CAD build for the part. Positions are in the model's coordinates, mm. A direction names the side the tool comes from. Round coordinates to 2 decimals unless told otherwise and drop trailing zeros.
from build123d import *

# Parameters (mm, degrees)
F0_R            = 19.05
F1_DEPTH        = 3.175
F3_DEPTH        = 6.35
F3_COPIES_COUNT = 16
F4_R            = 0.508
F5_R            = 6.35
F6_DEPTH        = 6.35


# Not quite as in the source:
# - a pattern or mirror of a feature is missing from the dataset's text; its kind, count and spacing are read off the source's solid


with BuildPart() as f1:
    # F0 (on Right) → F1 (new body, symmetric)
    with BuildSketch(Plane.YZ):
        Circle(F0_R)
    extrude(amount=F1_DEPTH, both=True)

    # F2 (on face) → F3 (cut, through all)
    with BuildSketch(Plane.YZ.offset(3.175)):
        with BuildLine():
            ThreePointArc((7.5322043505, 17.4976683482), (5.7520331342, 19.7340330411), (3.0490465261, 18.8044094638))
            Line((3.0490465261, 18.8044094638), (3.4766055202, 15.489636505))
            ThreePointArc((3.4766055202, 15.489636505), (4.4423475568, 15.2407733788), (5.3905576771, 14.931761883))
            Line((5.3905576771, 14.931761883), (7.5322043505, 17.4976683482))
        make_face()
    f3 = extrude(amount=-F3_DEPTH, mode=Mode.SUBTRACT)

    # F3_copies: F3 ×16 about axis
    f3_copies_axis = Axis((0, 0, 0), (1, 0, 0))
    for i in range(1, F3_COPIES_COUNT):
        add(f3.rotate(f3_copies_axis, i * 360 / F3_COPIES_COUNT), mode=Mode.SUBTRACT)

    # F4
    f4_edges = [f1.edges().sort_by_distance(p)[0] for p in [
        (0, 3.476606, 15.489637),
        (0, 5.390558, 14.931762),
        (0, 3.049047, 18.804409),
        (0, 7.532204, 17.497668),
        (0, 10.013088, 16.206189),
        (0, 9.139592, 12.980119),
        (0, 10.694364, 11.732272),
        (0, 13.654917, 13.283288),
        (0, 15.452727, 11.140724),
        (0, 13.411158, 8.494496),
        (0, 14.37005, 6.74665),
        (0, 17.698793, 7.046647),
        (0, 18.539829, 4.379184),
        (0, 15.640997, 2.715663),
        (0, 15.858026, 0.733912),
        (0, 19.048187, -0.262782),
        (0, 18.804409, -3.049047),
        (0, 15.489637, -3.476606),
        (0, 14.931762, -5.390558),
        (0, 17.497668, -7.532204),
        (0, 16.206189, -10.013088),
        (0, 12.980119, -9.139592),
        (0, 11.732272, -10.694364),
        (0, 13.283288, -13.654917),
        (0, 11.140724, -15.452727),
        (0, 8.494496, -13.411158),
        (0, 6.74665, -14.37005),
        (0, 7.046647, -17.698793),
        (0, 4.379184, -18.539829),
        (0, 2.715663, -15.640997),
        (0, 0.733912, -15.858026),
        (0, -0.262782, -19.048187),
        (0, -3.049047, -18.804409),
        (0, -3.476606, -15.489637),
        (0, -5.390558, -14.931762),
        (0, -7.532204, -17.497668),
        (0, -10.013088, -16.206189),
        (0, -9.139592, -12.980119),
        (0, -10.694364, -11.732272),
        (0, -13.654917, -13.283288),
        (0, -15.452727, -11.140724),
        (0, -13.411158, -8.494496),
        (0, -14.37005, -6.74665),
        (0, -17.698793, -7.046647),
        (0, -18.539829, -4.379184),
        (0, -15.640997, -2.715663),
        (0, -15.858026, -0.733912),
        (0, -19.048187, 0.262782),
        (0, -18.804409, 3.049047),
        (0, -15.489637, 3.476606),
        (0, -14.931762, 5.390558),
        (0, -17.497668, 7.532204),
        (0, -16.206189, 10.013088),
        (0, -12.980119, 9.139592),
        (0, -11.732272, 10.694364),
        (0, -13.283288, 13.654917),
        (0, -11.140724, 15.452727),
        (0, -8.494496, 13.411158),
        (0, -6.74665, 14.37005),
        (0, -7.046647, 17.698793),
        (0, -4.379184, 18.539829),
        (0, -2.715663, 15.640997),
        (0, -0.733912, 15.858026),
        (0, 0.262782, 19.048187),
    ]]
    fillet(f4_edges, radius=F4_R)

    # F5 (on face) → F6 (cut, through all)
    with BuildSketch(Plane.YZ.offset(3.175)):
        Circle(F5_R)
    extrude(amount=-F6_DEPTH, mode=Mode.SUBTRACT)


solid = f1.part
Item 1: Flat gauge pin, fed straight in: P1, Ø1, axis at x = -1, z = 3, coming from the -Y side. Where does the tip first touch, or does it go through?
Verdict:
P1: stops at y = -18.89
Item 2: 3-axis set-ups, long thin cutter, end or side, ignore diameter. For faces 1 (the flat face through (0.044, -6.894, 16.001)), 2 (the flat face through (0.04, 6.44, 16.19)), 3 (the flat face through (0.044, -14.434, -9.82)): which of +Z, -Z, +X, -X, +Y, -Y reach the whole face in a straight line?
Verdict:
face 1: +X, -X
face 2: +Z, +X, -X
face 3: +X, -X, -Y
Item 3: Wall check: L1, parallel to Y at x = -2.75, z = 16.5; L2, parallel to Y at x = -2.5, z = 16; L3, parallel to Y at x = -1, z = -13. Give the ranges that are in metal, low to high.
Verdict:
L1: y = -6.94 to -3.21, -0.53 to 3.35, 6.7 to 9.52
L2: y = -6.89 to -2.92, -0.74 to 3.41, 6.28 to 9.93
L3: y = -13.92 to -13.11, -9.25 to 12.94
Item 4: Mould opens along Z. For faces 4 (the flat face through (0.044, 17.093, 3.549)), 5 (the flat face through (3.175, 0, -8)), 6 (the flat face through (0.044, 3.262, 17.15)) say: released by +Z, released by -Z, zero draft, split by the parting line, or undercut.
Verdict:
face 4: undercut
face 5: zero draft
face 6: released by +Z
